```python
from build123d import *

# Parameters (mm, degrees)
F0_W         = 127
F0_H         = 76.2
F1_DEPTH     = 55
F2_R         = 5.08
F3_W         = 7
F3_H         = 14.3
F4_DEPTH     = 16.4
F5_DEPTH     = 25.4
F6_W         = 7
F6_H         = 14.3
F6_W_2       = 7.0104
F6_H_2       = 14.117781591
F7_DEPTH     = 16.4
F9_W         = 19.8135651034
F9_H         = 65.8797910702
F10_DEPTH    = 2.54
F11_T1_DEPTH = 87.8768363263
F11_T3_DEPTH = 41.8106103595
F12_DEPTH    = 1.524
F13_R        = 3
F13_R_2      = 1.8
F14_DEPTH    = 3.3
F15_DEPTH    = 11
F8_R         = 5.878920021
F16_DEPTH    = 1.016


# Not quite as in the source:
# - a fillet or chamfer that OpenCascade refuses, or shapes differently, is made with other operations: its cross-section is extruded or revolved along the edge and cut away or added


with BuildPart() as f1:
    # F0 (on Front) → F1 (new body)
    with BuildSketch(Plane.XZ):
        Rectangle(F0_W, F0_H)
    extrude(amount=F1_DEPTH)

    # F2
    f2_edges = [f1.edges().sort_by_distance(p)[0] for p in [
        (0, -55, -38.1),
        (0, 0, -38.1),
        (0, -55, 38.1),
        (0, 0, 38.1),
    ]]
    fillet(f2_edges, radius=F2_R)

    # F3 (on face) → F4 (cut)
    with BuildSketch(Plane.YZ.offset(63.5)):
        with Locations((-49.3123565018, 17.8676303864)):
            Rectangle(F3_W, F3_H)
        with Locations((-35.2098751962, 17.8676303864)):
            Rectangle(F3_W, F3_H)
        with Locations((-21.6830033958, 17.8676303864)):
            Rectangle(F3_W, F3_H)
        with Locations((-7.8683277741, 17.8676303864)):
            Rectangle(F3_W, F3_H)
    extrude(amount=-F4_DEPTH, mode=Mode.SUBTRACT)

    # F5 (cut): a face of the model
    f5_faces = [f1.faces().sort_by_distance(p)[0] for p in [
        (0, -55, 0),
    ]]
    extrude(f5_faces, amount=-F5_DEPTH, mode=Mode.SUBTRACT)

    # F6 (on face) → F7 (cut)
    with BuildSketch(Plane.YZ.offset(63.5)):
        with Locations((-21.6830033958, -17.639610437)):
            Rectangle(F6_W, F6_H)
        with Locations((-7.8631268428, -17.5485012325)):
            Rectangle(F6_W_2, F6_H_2)
    extrude(amount=-F7_DEPTH, mode=Mode.SUBTRACT)

    # F9 (on face) → F10 (join)
    with BuildSketch(Plane(origin=(-63.5, 0, 0), x_dir=(0, -1, 0), z_dir=(-1, 0, 0))):
        with Locations((14.9867825517, 0.0801044649)):
            Rectangle(F9_W, F9_H)
    extrude(amount=F10_DEPTH)

    # F11: fillet of radius 5.08 on 4 edges, made by hand

    # F11_s2 → F11_t1 (cut)
    with BuildSketch(Plane.XY.offset(-43.8583136983)):
        with BuildLine():
            ThreePointArc((-63.5, -24.8935651034), (-65.3594090512, -23.0341560522), (-66.04, -20.4941560522))
            Line((-66.04, -20.4941560522), (-66.04, -24.8935651034))
            Line((-66.04, -24.8935651034), (-63.5, -24.8935651034))
        make_face()
        with BuildLine():
            ThreePointArc((-63.5, -5.08), (-65.3594090512, -6.9394090512), (-66.04, -9.4794090512))
            Line((-66.04, -9.4794090512), (-66.04, -5.08))
            Line((-66.04, -5.08), (-63.5, -5.08))
        make_face()
    extrude(amount=F11_T1_DEPTH, mode=Mode.SUBTRACT)

    # F11_s4 → F11_t3 (cut)
    with BuildSketch(Plane.XZ.offset(-5.9185226281)):
        with BuildLine():
            ThreePointArc((-63.5, 33.02), (-65.3594090512, 31.1605909488), (-66.04, 28.6205909488))
            Line((-66.04, 28.6205909488), (-66.04, 33.02))
            Line((-66.04, 33.02), (-63.5, 33.02))
        make_face()
        with BuildLine():
            ThreePointArc((-63.5, -32.8597910702), (-65.3594090512, -31.000382019), (-66.04, -28.460382019))
            Line((-66.04, -28.460382019), (-66.04, -32.8597910702))
            Line((-66.04, -32.8597910702), (-63.5, -32.8597910702))
        make_face()
    extrude(amount=F11_T3_DEPTH, mode=Mode.SUBTRACT)

    # F12 (cut): a face of the model
    f12_faces = [f1.faces().sort_by_distance(p)[0] for p in [
        (-66.04, -14.9867825517, 0.0801044649),
    ]]
    extrude(f12_faces, amount=-F12_DEPTH, mode=Mode.SUBTRACT)

    # F13 (on face) → F14 (cut)
    with BuildSketch(Plane.YZ.offset(63.5)):
        with Locations((-14.8709248751, 33.3571620286)):
            Circle(F13_R)
        with Locations((-14.8709248751, 33.3571620286)):
            Circle(F13_R_2, mode=Mode.SUBTRACT)
    extrude(amount=-F14_DEPTH, mode=Mode.SUBTRACT)

    # F15 (cut): a face of the model
    f15_faces = [f1.faces().sort_by_distance(p)[0] for p in [
        (63.5, -14.8709248751, 33.3571620286),
    ]]
    extrude(f15_faces, amount=-F15_DEPTH, mode=Mode.SUBTRACT)

    # F8 (on face) → F16 (join)
    with BuildSketch(Plane.YZ.offset(63.5)):
        with Locations((-14.821995981, 0)):
            Circle(F8_R)
    extrude(amount=F16_DEPTH)


solid = f1.part
```
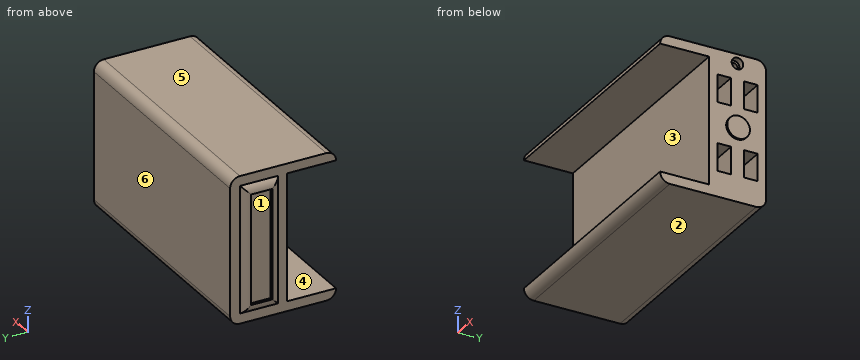
Work out the finished part from the listing and answer in its coordinate system (mm). Face numbers are marked on the shaded views. A direction names the side the tool comes from. Round coordinates to 2 decimals unless told otherwise and drop trailing zeros. Loops run counter-clockwise (first coordinate to the right, second up) from the corner with the lowest first, then second, coordinate; pieces in that order, holes last. Notation, with made-up numbers: M 57,85 L 67,85 A22 ccw 67,120 Z; hole C 44,53.25 d7. An arc over 180 degrees is marked long. One line per question, with ' | ' between items.
Q1. A tool of negligible diameter and unlimited length cuts with its end or side. For the marked faces 1, 2 and 3, from which of +Z, -Z, +X, -X, +Y, -Y can it reach the whole face along a straight path? Write none if from no direction.
Conclusion:
face 1: -X | face 2: -Z, +X, -X, +Y, -Y | face 3: +X, -X, -Y
Q2. Each of these flat-tipped pins is pushed along its axis until it touches: pin 1 Ø6.5 at (y, z) = (-15, 33.5) entering from +X; pin 2 Ø2 at (y, z) = (-22, 20) entering from +X; pin 3 Ø8 at (y, z) = (-14.87, 33.36) entering from -X. Where does it stop, or does it pass through?
Conclusion:
pin 1: stops at x = 63.5 | pin 2: stops at x = 47.1 | pin 3: stops at x = -65.99
Q3. The mould has two halves that part along Z. Classify the marked faces 4, 5 and 6: +Z half, -Z half, draft (parallel to the pull), parting line (faces both ways), or undercut.
Conclusion:
face 4: undercut | face 5: +Z half | face 6: draft
Q4. Find section A-A, the plane y = -35. Give the vertices of the cut face in (x, z).
Conclusion:
outline: M -63.5,-38.1 L 63.5,-38.1 L 63.5,-33.02 L -63.5,-33.02 Z; M -63.5,33.02 L 63.5,33.02 L 63.5,38.1 L -63.5,38.1 Z
Q5. Consider line 1 along Z through (x, y) = (-3, -48); line 2 along Y through (x, z) = (-27, 28); line 3 along X through (y, z) = (-29, -20.5). Determine where each line is inside the solid, lowest interval first. Write a range as from..to.
Conclusion:
line 1: z = -38.1..-33.02, 33.02..38.1 | line 2: y = -29.6..0 | line 3: x = -63.5..63.5
Q6. Find section C-C, the plane x = 43.5. Give the vertices of the cut face in (y, z), then the cut area to 3 significant figures.
Conclusion:
outline: M -55,-33.02 A5.08 ccw -49.92,-38.1 L -5.08,-38.1 A5.08 ccw 0,-33.02 L 0,33.02 A5.08 ccw -5.08,38.1 L -49.92,38.1 A5.08 ccw -55,33.02 L -29.6,33.02 L -29.6,-33.02 Z | area: 2,490 mm2
Q7. Find section D-D, the plane z = 0. Give the vertices of the cut face in (x, y).
Conclusion:
outline: M -66.04,-20.49 A5.08 ccw -63.5,-24.89 L -63.5,-29.6 L 63.5,-29.6 L 63.5,-20.7 L 64.52,-20.7 L 64.52,-8.94 L 63.5,-8.94 L 63.5,0 L -63.5,0 L -63.5,-5.08 A5.08 ccw -66.04,-9.48 L -64.52,-9.48 L -64.52,-20.49 Z
Q8. Find section B-B, the plane z = -16.5. Give the vertices of the cut face in (x, y).
Conclusion:
outline: M -66.04,-20.49 A5.08 ccw -63.5,-24.89 L -63.5,-29.6 L 63.5,-29.6 L 63.5,-25.18 L 47.1,-25.18 L 47.1,-18.18 L 63.5,-18.18 L 63.5,-11.37 L 47.1,-11.37 L 47.1,-4.36 L 63.5,-4.36 L 63.5,0 L -63.5,0 L -63.5,-5.08 A5.08 ccw -66.04,-9.48 L -64.52,-9.48 L -64.52,-20.49 Z
